```python
from build123d import *

# Parameters (mm, degrees)
BOSS_EXTRUDE1_DEPTH     = 29
CUT_EXTRUDE3_DEPTH      = 149.365258737
CUT_EXTRUDE3_DEPTH_BACK = 149.365258737


with BuildPart() as part:
    # Sketch2 → Boss-Extrude1 (new body)
    with BuildSketch(Plane(origin=(0, 0, 0), x_dir=(1, 0, 0), z_dir=(0, 1, 0))):
        with BuildLine():
            Line((-23.389824888, -46), (23.389824888, -46))
            ThreePointArc((23.389824888, -46), (29.600414922, -48.162361872), (33.125096338, -53.714285714))
            ThreePointArc((33.125096338, -53.714285714), (90.695873622, -83.293048719), (110.70300535, -21.738095238))
            ThreePointArc((110.70300535, -21.738095238), (104.55417528, 0), (110.70300535, 21.738095238))
            ThreePointArc((110.70300535, 21.738095238), (90.695873622, 83.293048719), (33.125096338, 53.714285714))
            ThreePointArc((33.125096338, 53.714285714), (29.600414922, 48.162361872), (23.389824888, 46))
            Line((23.389824888, 46), (-23.389824888, 46))
            ThreePointArc((-23.389824888, 46), (-29.600414922, 48.162361872), (-33.125096338, 53.714285714))
            ThreePointArc((-33.125096338, 53.714285714), (-90.695873622, 83.293048719), (-110.70300535, 21.738095238))
            ThreePointArc((-110.70300535, 21.738095238), (-104.55417528, 0), (-110.70300535, -21.738095238))
            ThreePointArc((-110.70300535, -21.738095238), (-90.695873622, -83.293048719), (-33.125096338, -53.714285714))
            ThreePointArc((-33.125096338, -53.714285714), (-29.600414922, -48.162361872), (-23.389824888, -46))
        make_face()
    extrude(amount=BOSS_EXTRUDE1_DEPTH)

    # Sketch4 → Cut-Extrude3 (cut, two sides: drawn at the far end of the back side and taken through both)
    with BuildSketch(Plane.XY.offset(-CUT_EXTRUDE3_DEPTH_BACK)):
        with BuildLine():
            Line((-597.255249838, 23), (-117, 23))
            Line((-117, 23), (-35.764946788, 23))
            ThreePointArc((-35.764946788, 23), (-32.942865818, 22.127451877), (-31.105745429, 19.814343599))
            Line((-31.105745429, 19.814343599), (-26.432815133, 7.814343599))
            ThreePointArc((-26.432815133, 7.814343599), (-22.758574356, 3.188127043), (-17.114412415, 1.443030797))
            Line((-17.114412415, 1.443030797), (17.114412415, 1.443030797))
            ThreePointArc((17.114412415, 1.443030797), (22.758574356, 3.188127043), (26.432815133, 7.814343599))
            Line((26.432815133, 7.814343599), (31.105745429, 19.814343599))
            ThreePointArc((31.105745429, 19.814343599), (32.942865818, 22.127451877), (35.764946788, 23))
            Line((35.764946788, 23), (117, 23))
            Line((117, 23), (597.255249838, 23))
            Line((597.255249838, 23), (597.255249838, -937.510499676))
            Line((597.255249838, -937.510499676), (-597.255249838, -937.510499676))
            Line((-597.255249838, -937.510499676), (-597.255249838, 23))
        make_face()
    extrude(amount=CUT_EXTRUDE3_DEPTH + CUT_EXTRUDE3_DEPTH_BACK, mode=Mode.SUBTRACT)


solid = part.part
```
For this review, take the finished solid that the model builds, in its own axes (mm). A direction names the side the tool comes from. Coordinates: 2 decimals unless noted, no trailing zeros. Write each loop counter-clockwise with the first axis right and the second up, starting at its lowest first coordinate (ties: lowest second). Pieces come first, ordered by that corner, then holes.
(1) Add section C-C on z = 1. Give the boundary of the cut face in (x, y), then the cut area to 3 significant figures.
(2) Add section B-B on x = -4. Give the boundary of the cut face in (y, z), then the cut area to 3 significant figures.
(3) Tool access review of faces 1 (the face through (-77, 23, -1)), 2 (the face through (76, 23, -1)), 3 (the face through (-28.45, 18.967, 47.375)): name each direction out of +Z, -Z, +X, -X, +Y, -Y from which nothing blocks a thin tool from reaching the whole face with its end or side.
(4) Wall thickness on probe 1 along X at (y, z) = (25, 62.5); probe 2 along Y at (x, z) = (-37, -6); probe 3 along Z at (x, y) = (-21.5, 10.25): over which ranges is each line inside the solid? List them lowest first.
(5) Add section A-A on z = 28.5. Give the boundary of the cut face in (x, y), then the cut area to 3 significant figures.
(6) For pin 1 Ø12 at (x, y) = (-62, 26) entering from +Z; pin 2 Ø3 at (y, z) = (14, 40) entering from +X; pin 3 Ø24.5 at (x, z) = (90.5, -27.5) entering from -Y, all flat-tipped, find the tip position at first contact; note any pin that passes through.
(7) The part is to be moulded in two halves that separate along X. For faces 4 (the face through (91.64, 25.58, -82.89)), 5 (the face through (32.9, 22.1, -0.9)), 6 (the face through (-22.828, 3.236, -0.651)), say which applies: +X half, -X half, draft (parallel to the pull), parting line (faces both ways), or undercut.
(8) Add section D-D on x = -74.5. Give the boundary of the cut face in (y, z), then the cut area to 3 significant figures.
Answer sheet:
1. outline: (-104.57, 23) - (-35.76, 23) arc R5 cw to (-31.11, 19.81) - (-26.43, 7.81) arc R10 ccw to (-17.11, 1.44) - (17.11, 1.44) arc R10 ccw to (26.43, 7.81) - (31.11, 19.81) arc R5 cw to (35.76, 23) - (104.57, 23) - (104.57, 29) - (-104.57, 29) - close
1. area: 2,460 mm2
2. outline: (1.44, -46) - (29, -46) - (29, 46) - (1.44, 46) - close
2. area: 2,540 mm2
3. face 1: +Z, -Z, -X, -Y
3. face 2: +Z, -Z, +X, -Y
3. face 3: +Z, +Y, -Y
4. probe 1: x = -112.76 to -36.24, 36.24 to 112.76
4. probe 2: y = 23 to 29
4. probe 3: z = -46 to 46
5. outline: (-114.07, 23) - (-35.76, 23) arc R5 cw to (-31.11, 19.81) - (-26.43, 7.81) arc R10 ccw to (-17.11, 1.44) - (17.11, 1.44) arc R10 ccw to (26.43, 7.81) - (31.11, 19.81) arc R5 cw to (35.76, 23) - (114.07, 23) - (114.07, 29) - (-114.07, 29) - close
5. area: 2,570 mm2
6. pin 1: stops at z = 86
6. pin 2: stops at x = 29.43
6. pin 3: stops at y = 23
7. face 4: undercut
7. face 5: +X half
7. face 6: -X half
8. outline: (23, -86.5) - (29, -86.5) - (29, 86.5) - (23, 86.5) - close
8. area: 1,040 mm2
